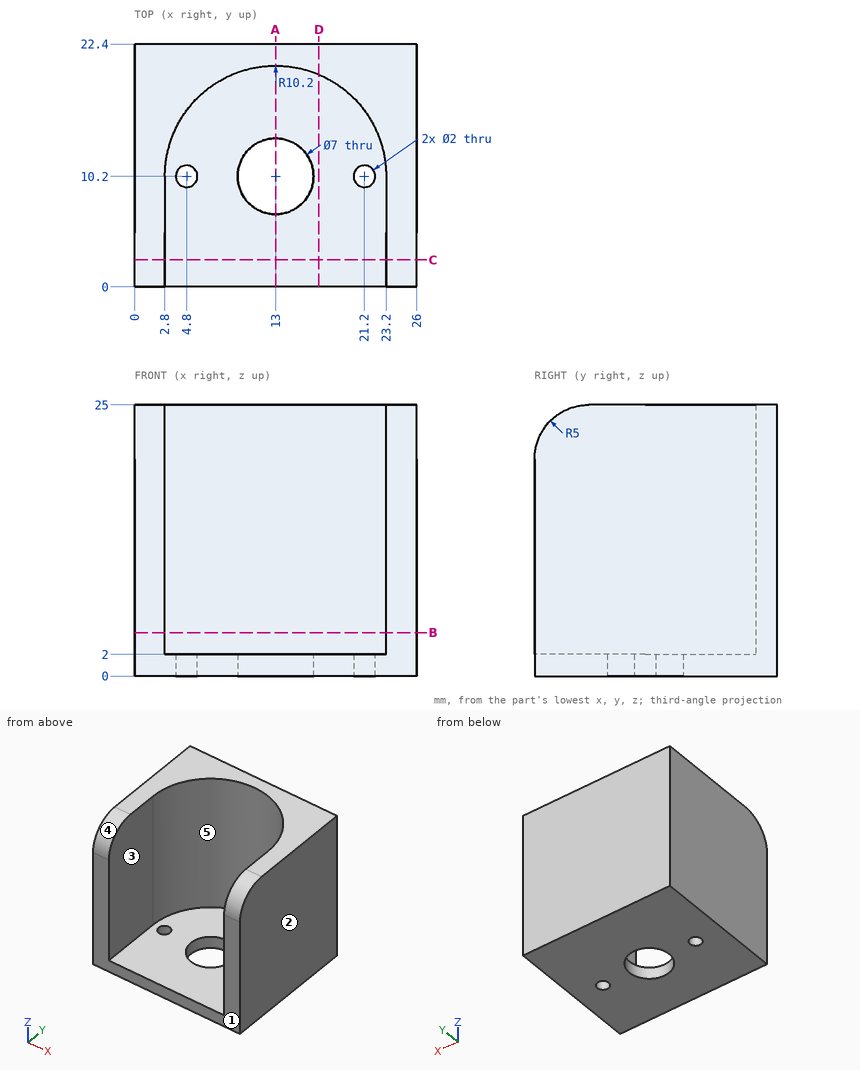
The drawing under review shows one solid part. Ordinate dimensions are in mm from its lowest x, y, z. A direction names the side the tool comes from. Coordinates: 2 decimals unless noted, no trailing zeros. Order: outer loops, then holes, each group sorted by start corner. A loop starts at its lowest first (then second) coordinate and runs counter-clockwise, first axis right, second up. Notation, with made-up numbers: (-14, -8.5) -> (-1, -8.5) arc R20 cw to (-1, 20.5) -> close; hole circle Ø9 at (9.25, -38.5). An arc over 180 degrees is marked (long way). Use CSV: the item, a comma, the result in double quotes. Start each with the question number.
Item 1: Insertion check: pin 1 (1.8 mm diameter, centred on x = 4.8, y = 10.2, fed in from +Z); pin 2 (4 mm diameter, centred on x = 15, y = 2.5, fed in from +Z). Each pin has a flat end and moves straight along its axis. Give the tip position at first contact, or say it passes through.
Item 2: Wall thickness on probe 1 along X at (y, z) = (2.5, 7.5); probe 2 along Y at (x, z) = (21.2, 1.1); probe 3 along Z at (x, y) = (19, 5.5): over which ranges is each line inside the solid? List them lowest first.
Item 3: We need section B-B, the plane z = 4. Give the boundary of the cut face in (x, y).
Item 4: We need section C-C, the plane y = 2.5. Give the boundary of the cut face in (x, z), then the cut area to 3 significant figures.
Item 5: We need section D-D, the plane x = 17. Give the boundary of the cut face in (y, z).
Item 6: Draft analysis for pull direction X (two halves, no side actions). For the marked faces 1, 2 and 3, state which applies: pulls with the +X half, pulls with the -X half, needs draft (parallel to the pull), parting line crosses it, or undercut.
Item 7: For the marked faces 4 and 5, list the 3-axis set-ups (+Z, -Z, +X, -X, +Y, -Y) from which the entire face can be reached by the end or side of a thin tool; tool diameter is ignored.
Item 8: We need section A-A, the plane x = 13. Give the boundary of the cut face in (y, z), then the cut area to 3 significant figures.
Derived:
1,pin 1,"passes through"
1,pin 2,"stops at z = 2"
2,probe 1,"x = 0 to 2.8, 23.2 to 26"
2,probe 2,"y = 0 to 9.2, 11.2 to 22.4"
2,probe 3,"z = 0 to 2"
3,outline,"(0, 0) -> (2.8, 0) -> (2.8, 10.2) arc R10.2 cw to (23.2, 10.2) -> (23.2, 0) -> (26, 0) -> (26, 22.4) -> (0, 22.4) -> close"
4,outline,"(0, 0) -> (26, 0) -> (26, 24.33) -> (23.2, 24.33) -> (23.2, 2) -> (2.8, 2) -> (2.8, 24.33) -> (0, 24.33) -> close"
4,area,"177 mm^2"
5,outline,"(0, 0) -> (22.4, 0) -> (22.4, 25) -> (19.58, 25) -> (19.58, 2) -> (0, 2) -> close"
6,face 1,"needs draft"
6,face 2,"pulls with the +X half"
6,face 3,"undercut"
7,face 4,"+Z, +X, -X, -Y"
7,face 5,"+Z, -Y"
8,outline,"(0, 0) -> (6.7, 0) -> (6.7, 2) -> (0, 2) -> close; (13.7, 0) -> (22.4, 0) -> (22.4, 25) -> (20.4, 25) -> (20.4, 2) -> (13.7, 2) -> close"
8,area,"76.8 mm^2"
